Read the model definition and answer for the solid it produces. Units are mm, in the model's axes. A direction names the side the tool comes from. Coordinates: 2 decimals unless noted, no trailing zeros. Write each loop counter-clockwise with the first axis right and the second up, starting at its lowest first coordinate (ties: lowest second). Pieces come first, ordered by that corner, then holes. Notation, with made-up numbers: (-21.5, 83.25) -> (9.5, 83.25) arc R20 cw to (9.5, 116.25) -> close; hole circle Ø2 at (82.5, 62). An arc over 180 degrees is marked (long way). Return JSON: item names as keys, results as strings.
from build123d import *

# Parameters (mm, degrees)
SKETCH1_R           = 19.05
SKETCH1_R_2         = 7.62
BOSS_EXTRUDE1_DEPTH = 83.348208
SKETCH3_R           = 11.1125
CUT_EXTRUDE2_DEPTH  = 5.5562754
CUT_EXTRUDE3_START  = -5.5562754
SKETCH4_R           = 11.1125
CUT_EXTRUDE3_DEPTH  = 5.5562754
SKETCH13_R          = 1.75
CUT_EXTRUDE4_DEPTH  = 13
CIRPATTERN2_COUNT   = 4
CUT_EXTRUDE6_START  = -13
SKETCH19_R          = 1.75
CUT_EXTRUDE6_DEPTH  = 13
CIRPATTERN4_COUNT   = 4


with BuildPart() as part:
    # Sketch1 → Boss-Extrude1 (new body)
    with BuildSketch(Plane(origin=(0, 0, 0), x_dir=(1, 0, 0), z_dir=(0, 1, 0))):
        with Locations(Location((0, 0, 0), (0, 0, 270))):
            Circle(SKETCH1_R)
        with Locations(Location((0, 0, 0), (0, 0, 270))):
            Circle(SKETCH1_R_2, mode=Mode.SUBTRACT)
    extrude(amount=BOSS_EXTRUDE1_DEPTH)

    # Sketch3 → Cut-Extrude2 (cut)
    with BuildSketch(Plane(origin=(0, 83.348208, 0), x_dir=(1, 0, 0), z_dir=(0, 1, 0))):
        with Locations(Location((0, 0, 0), (0, 0, 270))):
            Circle(SKETCH3_R)
    extrude(amount=-CUT_EXTRUDE2_DEPTH, mode=Mode.SUBTRACT)

    # Sketch4 → Cut-Extrude3 (cut)
    with BuildSketch(Plane.XZ.offset(CUT_EXTRUDE3_START)):
        with Locations(Location((0, 0, 0), (0, 0, 90))):
            Circle(SKETCH4_R)
    extrude(amount=CUT_EXTRUDE3_DEPTH, mode=Mode.SUBTRACT)

    # Sketch13 → Cut-Extrude4 (cut)
    with BuildSketch(Plane(origin=(0, 83.348208, 0), x_dir=(1, 0, 0), z_dir=(0, 1, 0))):
        with Locations(Location((0, 15, 0), (0, 0, 270))):
            Circle(SKETCH13_R)
    cut_extrude4 = extrude(amount=-CUT_EXTRUDE4_DEPTH, mode=Mode.SUBTRACT)

    # CirPattern2: Cut-Extrude4 ×4 about axis
    cirpattern2_axis = Axis((0, 0, 0), (0, 1, 0))
    for i in range(1, CIRPATTERN2_COUNT):
        add(cut_extrude4.rotate(cirpattern2_axis, i * 360 / CIRPATTERN2_COUNT), mode=Mode.SUBTRACT)

    # Sketch19 → Cut-Extrude6 (cut)
    with BuildSketch(Plane.XZ.offset(CUT_EXTRUDE6_START)):
        with Locations(Location((0, 15, 0), (0, 0, 90))):
            Circle(SKETCH19_R)
    cut_extrude6 = extrude(amount=CUT_EXTRUDE6_DEPTH, mode=Mode.SUBTRACT)

    # CirPattern4: Cut-Extrude6 ×4 about axis
    cirpattern4_axis = Axis((0, 0, 0), (0, 1, 0))
    for i in range(1, CIRPATTERN4_COUNT):
        add(cut_extrude6.rotate(cirpattern4_axis, i * 360 / CIRPATTERN4_COUNT), mode=Mode.SUBTRACT)


solid = part.part
1. Flat-ended cylindrical pins translate along their axes: pin 1 Ø1.8 at (x, z) = (0, 15) entering from -Y; pin 2 Ø3 at (x, y) = (-14, 27.5) entering from +Z; pin 3 Ø5 at (y, z) = (41, 15) entering from +X. Find the tip coordinate at first contact, or state that the pin passes through.
Taken from the geometry:
{"pin 1": "stops at y = 13", "pin 2": "stops at z = 14.38", "pin 3": "stops at x = 14.38"}
2. The part is cut by section C-C (y = 49). Determine the outline of the cut face in (x, z).
Taken from the geometry:
{"outline": "circle Ø38.1 at (0, 0); hole circle Ø15.24 at (0, 0)"}
3. A tool of negligible diameter and unlimited length cuts with its end or side. For faces 5 (the face through (7.555, 41.168, -0.992)), 6 (the face through (-9.37, 2.817, 5.974)), 7 (the face through (8, 77.792, 2)), from which of +Z, -Z, +X, -X, +Y, -Y can it reach the whole face along a straight path? Write none if from no direction.
Taken from the geometry:
{"face 5": "+Y, -Y", "face 6": "-Y", "face 7": "+Y"}
4. Consider L1, parallel to X at y = 21, z = 0; L2, parallel to Y at x = 10.5, z = -2; L3, parallel to Z at x = -1, y = 26. Determine where each line is inside the solid, lowest interval first.
Taken from the geometry:
{"L1": "x = -19.05 to -7.62, 7.62 to 19.05", "L2": "y = 5.56 to 77.79", "L3": "z = -19.02 to -7.55, 7.55 to 19.02"}
5. For a pull along X with two mould halves and no side action, classify faces 1 (the face through (-11.59, 41.09, -15.12)), 2 (the face through (-0.526, 76.939, 13.331)), 3 (the face through (-8, 0, 8)), 4 (the face through (-15, 70.348, 0)) as +X half, -X half, draft (parallel to the pull), parting line (faces both ways), or undercut.
Taken from the geometry:
{"face 1": "parting line", "face 2": "undercut", "face 3": "draft", "face 4": "undercut"}
6. The part is cut by section D-D (x = -15.5). Determine the outline of the cut face in (y, z).
Taken from the geometry:
{"outline": "(0, -11.07) -> (83.35, -11.07) -> (83.35, -1.68) -> (70.35, -1.68) -> (70.35, 1.68) -> (83.35, 1.68) -> (83.35, 11.07) -> (0, 11.07) -> (0, 1.68) -> (13, 1.68) -> (13, -1.68) -> (0, -1.68) -> close"}
